from build123d import *

# Parameters (mm, degrees)
F0_W      = 85
F0_H      = 74
F0_R      = 2.1
F1_DEPTH  = 12
F2_W      = 80.5
F2_H      = 70
F2_R      = 2.1
F3_DEPTH  = 10
F4_W      = 6
F4_H      = 42
F4_W_2    = 49.8
F4_H_2    = 8
F4_W_3    = 24.7
F4_H_3    = 20
F5_DEPTH  = 7
F6_R      = 1.45
F7_DEPTH  = 3.5
F8_W      = 2.25
F8_H      = 38
F9_DEPTH  = 2
F11_DEPTH = 10
F12_W     = 2.25
F12_H     = 15
F13_DEPTH = 2
F14_R     = 12
F15_R     = 3
F17_DEPTH = 2
F19_DEPTH = 2
F21_DEPTH = 2
F22_R     = 4
F23_R     = 2
F6_R_2    = 1.4
F24_DEPTH = 9
F25_W     = 6
F25_H     = 5
F25_R     = 1.4
F26_DEPTH = 3
F27_W     = 5
F27_H     = 8
F28_DEPTH = 1


with BuildPart() as f1:
    # F0 (on Top) → F1 (new body)
    with BuildSketch(Plane.XY):
        Rectangle(F0_W, F0_H)
        with Locations((-30, -27)):
            Circle(F0_R, mode=Mode.SUBTRACT)
        with Locations((30, -27)):
            Circle(F0_R, mode=Mode.SUBTRACT)
        with Locations((-30, 8)):
            Circle(F0_R, mode=Mode.SUBTRACT)
        with Locations((30, 8)):
            Circle(F0_R, mode=Mode.SUBTRACT)
    extrude(amount=F1_DEPTH)

    # F2 (on face) → F3 (cut)
    with BuildSketch(Plane.XY.offset(12)):
        Rectangle(F2_W, F2_H)
        with Locations((-30, -27)):
            Circle(F2_R, mode=Mode.SUBTRACT)
        with Locations((30, -27)):
            Circle(F2_R, mode=Mode.SUBTRACT)
        with Locations((-30, 8)):
            Circle(F2_R, mode=Mode.SUBTRACT)
        with Locations((30, 8)):
            Circle(F2_R, mode=Mode.SUBTRACT)
    extrude(amount=-F3_DEPTH, mode=Mode.SUBTRACT)

    # F4 (on face) → F5 (join)
    with BuildSketch(Plane.XY.offset(2)):
        with Locations((12.55, 14)):
            Rectangle(F4_W, F4_H)
        with Locations((-15.35, -11)):
            Rectangle(F4_W_2, F4_H_2)
        with Locations((12.55, -11)):
            Rectangle(F4_W, F4_H_2)
        with Locations((27.9, -11)):
            Rectangle(F4_W_3, F4_H_2)
        with Locations((12.55, -25)):
            Rectangle(F4_W, F4_H_3)
    extrude(amount=F5_DEPTH)

    # F6 (on face) → F7 (join)
    with BuildSketch(Plane.XY.offset(9)):
        with Locations((11.05, -24.1)):
            Circle(F6_R)
    extrude(amount=F7_DEPTH)

    # F8 (on face) → F9 (cut)
    with BuildSketch(Plane.XY.offset(12)):
        with Locations((-41.375, 5)):
            Rectangle(F8_W, F8_H)
    extrude(amount=-F9_DEPTH, mode=Mode.SUBTRACT)

    # F10 (on face) → F11 (cut, through all)
    with BuildSketch(Plane.XY.offset(12)):
        Polygon((-42.5, 37), (-42.5, 24), (-40.25, 24), (-40.25, 35), (-22.5, 35), (-22.5, 37), align=None)
        Polygon((42.5, 37), (22.5, 37), (22.5, 35), (40.25, 35), (40.25, 17), (42.5, 17), align=None)
        Polygon((42.5, -37), (42.5, -22), (40.25, -22), (40.25, -35), (22.5, -35), (22.5, -37), align=None)
        Polygon((-42.5, -37), (-22.5, -37), (-22.5, -35), (-40.25, -35), (-40.25, -22), (-42.5, -22), align=None)
    extrude(amount=-F11_DEPTH, mode=Mode.SUBTRACT)

    # F12 (on face) → F13 (cut)
    with BuildSketch(Plane.XY.offset(12)):
        with Locations((41.375, -12)):
            Rectangle(F12_W, F12_H)
    extrude(amount=-F13_DEPTH, mode=Mode.SUBTRACT)

    # F14
    f14_edges = [f1.edges().sort_by_distance(p)[0] for p in [
        (-42.5, 37, 1),
        (-42.5, -37, 1),
        (42.5, -37, 1),
        (42.5, 37, 1),
    ]]
    fillet(f14_edges, radius=F14_R)

    # F15
    f15_edges = [f1.edges().sort_by_distance(p)[0] for p in [
        (9.55, -7, 5.5),
        (9.55, -15, 5.5),
        (15.55, -15, 5.5),
        (15.55, -7, 5.5),
        (-40.25, -7, 5.5),
        (-40.25, -15, 5.5),
        (9.55, 35, 5.5),
        (15.55, 35, 5.5),
        (9.55, -35, 5.5),
        (40.25, -15, 5.5),
        (15.55, -35, 5.5),
    ]]
    fillet(f15_edges, radius=F15_R)

    # F16 (on face) → F17 (cut, through all)
    with BuildSketch(Plane.XY.offset(2)):
        with BuildLine():
            ThreePointArc((9.55, -18), (8.6713203436, -15.8786796564), (6.55, -15))
            Line((6.55, -15), (-22.5, -15))
            Line((-22.5, -15), (-22.5, -35))
            Line((-22.5, -35), (6.55, -35))
            ThreePointArc((6.55, -35), (8.6713203436, -34.1213203436), (9.55, -32))
            Line((9.55, -32), (9.55, -18))
        make_face()
    extrude(amount=-F17_DEPTH, mode=Mode.SUBTRACT)

    # F18 (on face) → F19 (cut, through all)
    with BuildSketch(Plane.XY.offset(2)):
        with BuildLine():
            Line((-22.5, 35), (-22.5, -7))
            Line((-22.5, -7), (6.55, -7))
            ThreePointArc((6.55, -7), (8.6713203436, -6.1213203436), (9.55, -4))
            Line((9.55, -4), (9.55, 32))
            ThreePointArc((9.55, 32), (8.6713203436, 34.1213203436), (6.55, 35))
            Line((6.55, 35), (-22.5, 35))
        make_face()
    extrude(amount=-F19_DEPTH, mode=Mode.SUBTRACT)

    # F20 (on face) → F21 (cut, through all)
    with BuildSketch(Plane.XY.offset(2)):
        with BuildLine():
            ThreePointArc((18.55, 35), (16.4286796564, 34.1213203436), (15.55, 32))
            Line((15.55, 32), (15.55, 17))
            Line((15.55, 17), (40.25, 17))
            Line((40.25, 17), (42.5, 17))
            Line((42.5, 17), (42.5, 25))
            ThreePointArc((42.5, 25), (38.9852813742, 33.4852813742), (30.5, 37))
            Line((30.5, 37), (22.5, 37))
            Line((22.5, 37), (22.5, 35))
            Line((22.5, 35), (18.55, 35))
        make_face()
    extrude(amount=-F21_DEPTH, mode=Mode.SUBTRACT)

    # F22
    f22_edges = [f1.edges().sort_by_distance(p)[0] for p in [
        (-22.5, 35, 1),
        (-22.5, -7, 1),
        (15.55, 17, 1),
        (-22.5, -15, 1),
        (-22.5, -35, 1),
    ]]
    fillet(f22_edges, radius=F22_R)

    # F23
    f23_edges = [f1.edges().sort_by_distance(p)[0] for p in [
        (-22.5, -36, 12),
        (22.5, -36, 12),
        (-41.375, -22, 12),
        (-22.5, 36, 12),
        (-22.5, 36, 2),
        (22.5, 36, 12),
        (41.375, 17, 12),
        (-41.375, 24, 10),
        (-22.5, -36, 2),
        (22.5, -36, 2),
        (41.375, -22, 2),
        (-41.375, -22, 2),
        (-41.375, 24, 2),
    ]]
    fillet(f23_edges, radius=F23_R)

    # F6 (on face) → F24 (cut, through all)
    with BuildSketch(Plane.XY.offset(9)):
        with Locations((12.35, 24.2)):
            Circle(F6_R_2)
    extrude(amount=-F24_DEPTH, mode=Mode.SUBTRACT)

    # F25 (on face) → F26 (cut)
    with BuildSketch(Plane(origin=(0, 0, 0), x_dir=(1, 0, 0), z_dir=(0, 0, -1))):
        with Locations((12.55, -24.2)):
            Rectangle(F25_W, F25_H)
        with Locations((12.35, -24.2)):
            Circle(F25_R, mode=Mode.SUBTRACT)
    extrude(amount=-F26_DEPTH, mode=Mode.SUBTRACT)

    # F27 (on face) → F28 (join, through all)
    with BuildSketch(Plane.XY.offset(9)):
        with Locations((37.75, -11)):
            Rectangle(F27_W, F27_H)
    extrude(amount=F28_DEPTH)


solid = f1.part
Build history of the part. All positions in model axes, mm. A direction names the side the tool comes from. Coordinates: 2 decimals unless noted, no trailing zeros. Write each loop counter-clockwise with the first axis right and the second up, starting at its lowest first coordinate (ties: lowest second). Pieces come first, ordered by that corner, then holes. Notation, with made-up numbers: (-14.75, 37.5) -> (6.25, 37.5) arc R21 cw to (6.25, 44.5) -> close; hole circle Ø2 at (-1.75, -34.75). An arc over 180 degrees is marked (long way). Use CSV: the item, a comma, the result in double quotes. Start each with the question number.
Q1. Flat gauge pins, fed straight in: pin 1 Ø5.5 at (x, y) = (30, -27) entering from +Z; pin 2 Ø4 at (x, y) = (-30, -27) entering from -Z; pin 3 Ø1.1 at (x, z) = (41.5, 7.5) entering from -Y; pin 4 Ø6 at (x, z) = (-28, 8) entering from +Y. Where does each tip first touch, or does it go through?
Q2. Cut at D-D, the plane y = -27. List the corners of the cut face in (x, z).
Q3. 3-axis set-ups, long thin cutter, end or side, ignore diameter. For faces 4 (the cylindrical face through (-21.359, -16.203, 0.986)), 5 (the flat face through (-31, 15, 2)), 6 (the flat face through (41, -22, 8)), 7 (the flat face through (41, -19.5, 11)): which of +Z, -Z, +X, -X, +Y, -Y reach the whole face in a straight line?
Q4. Cut at C-C, the plane y = -11. List the corners of the cut face in (x, z), then the cut area to 4 significant figures.
Q5. Cut at A-A, the plane y = 1. List the corners of the cut face in (x, z), then the cut area to 3 significant figures.
Q6. Pull direction X, two halves, no side cores. Call faces 1 (the cylindrical face through (-41.39, -22.6, 2.57)), 2 (the cylindrical face through (-21.9, -35.99, 11.43)), 3 (the cylindrical face through (27.9, -26.91, 0.99)): released by +X, released by -X, zero draft, split by the parting line, or undercut.
Q7. Cut at B-B, the plane x = -1. List the corners of the cut face in (y, z).
Q8. Drill centre lines: probe 1 along X at (y, z) = (1, 8.5); probe 2 along Y at (x, z) = (30, 1.3); probe 3 along Y at (x, z) = (-30, 0.9). Where is each one in solid material? Low to high.
Checked values:
1,pin 1,"stops at z = 2"
1,pin 2,"passes through"
1,pin 3,"stops at y = -22"
1,pin 4,"stops at y = -7"
2,outline,"(-42.33, 0) -> (-32.1, 0) -> (-32.1, 2) -> (-42.33, 2) -> close; (-27.9, 0) -> (-22.5, 0) -> (-22.5, 2) -> (-27.9, 2) -> close; (9.55, 0) -> (27.9, 0) -> (27.9, 2) -> (15.55, 2) -> (15.55, 9) -> (9.55, 9) -> close; (32.1, 0) -> (42.33, 0) -> (42.33, 2) -> (32.1, 2) -> close"
3,face 4,"+Z, -Z"
3,face 5,"+Z"
3,face 6,"+Z, +X, -Y"
3,face 7,"+Z, +X"
4,outline,"(-42.5, 0) -> (42.5, 0) -> (42.5, 10) -> (35.25, 10) -> (35.25, 9) -> (-40.25, 9) -> (-40.25, 10) -> (-42.5, 10) -> close"
4,area,"774.5 mm²"
5,outline,"(-42.5, 0) -> (-22.5, 0) -> (-22.5, 2) -> (-40.25, 2) -> (-40.25, 10) -> (-42.5, 10) -> close; (9.55, 0) -> (42.5, 0) -> (42.5, 12) -> (40.25, 12) -> (40.25, 2) -> (15.55, 2) -> (15.55, 9) -> (9.55, 9) -> close"
5,area,"188 mm²"
6,face 1,"zero draft"
6,face 2,"released by -X"
6,face 3,"undercut"
7,outline,"(-37, 0) -> (-35, 0) -> (-35, 12) -> (-37, 12) -> close; (-15, 0) -> (-7, 0) -> (-7, 9) -> (-15, 9) -> close; (35, 0) -> (37, 0) -> (37, 12) -> (35, 12) -> close"
8,probe 1,"x = -42.5 to -40.25, 9.55 to 15.55, 40.25 to 42.5"
8,probe 2,"y = -37 to -29.1, -24.9 to 5.9, 10.1 to 17"
8,probe 3,"y = -37 to -29.1, -24.9 to 5.9, 10.1 to 37"
